```python
from build123d import *
from build123d.topology import SkipClean

# Parameters (mm, degrees)
SKETCH1_R           = 15.5
SKETCH1_R_2         = 12
BOSS_EXTRUDE1_DEPTH = 4
BOSS_EXTRUDE2_START = 13
SKETCH2_R           = 14
SKETCH2_R_2         = 12
BOSS_EXTRUDE2_DEPTH = 13
BOSS_EXTRUDE3_DEPTH = 0.5
CIRPATTERN1_COUNT   = 4
BOSS_EXTRUDE4_START = -4
SKETCH4_R           = 1.5
BOSS_EXTRUDE4_DEPTH = 4
CIRPATTERN2_COUNT   = 4
SKETCH5_R           = 12
BOSS_EXTRUDE5_DEPTH = 2


with BuildPart() as part:
    # Sketch1 → Boss-Extrude1 (new body)
    with BuildSketch(Plane(origin=(0, 0, 0), x_dir=(1, 0, 0), z_dir=(0, 1, 0))):
        with Locations(Location((0, 0, 0), (0, 0, 270))):
            Circle(SKETCH1_R)
        with Locations(Location((0, 0, 0), (0, 0, 270))):
            Circle(SKETCH1_R_2, mode=Mode.SUBTRACT)
    extrude(amount=BOSS_EXTRUDE1_DEPTH)

    # Sketch2 → Boss-Extrude2 (add)
    with SkipClean():  # the faces are left unmerged after this step: merging them gives an invalid solid
        with BuildSketch(Plane.XZ.offset(BOSS_EXTRUDE2_START)):
            with Locations(Location((0, 0, 0), (0, 0, 90))):
                Circle(SKETCH2_R)
            with Locations(Location((0, 0, 0), (0, 0, 270))):
                Circle(SKETCH2_R_2, mode=Mode.SUBTRACT)
        extrude(amount=-BOSS_EXTRUDE2_DEPTH)

    # Sketch3 → Boss-Extrude3 (add, symmetric)
    with SkipClean():  # the faces are left unmerged after this step: merging them gives an invalid solid
        with BuildSketch(Plane(origin=(0, 0, 0), x_dir=(0, 0, -1), z_dir=(1, 0, 0))):
            Polygon((-12, 0), (-3.5, -11), (3.5, -11), (12, 0), (12, -13), (-12, -13), align=None)
        boss_extrude3 = extrude(amount=BOSS_EXTRUDE3_DEPTH, both=True)

    # CirPattern1: Boss-Extrude3 ×4 about axis
    with SkipClean():  # the faces are left unmerged after this step: merging them gives an invalid solid
        cirpattern1_axis = Axis((0, 0, 0), (0, 1, 0))
        for i in range(1, CIRPATTERN1_COUNT):
            add(boss_extrude3.rotate(cirpattern1_axis, i * 360 / CIRPATTERN1_COUNT))

    # Sketch4 → Boss-Extrude4 (add)
    with SkipClean():  # the faces are left unmerged after this step: merging them gives an invalid solid
        with BuildSketch(Plane(origin=(0, 4, 0), x_dir=(1, 0, 0), z_dir=(0, 1, 0)).offset(BOSS_EXTRUDE4_START)):
            with BuildLine():
                Line((-2.785012774, 19.115214709), (-4.5, 14.832396974))
                ThreePointArc((-4.5, 14.832396974), (0, 15.5), (4.5, 14.832396974))
                Line((4.5, 14.832396974), (2.785012774, 19.115214709))
                ThreePointArc((2.785012774, 19.115214709), (0, 21), (-2.785012774, 19.115214709))
            make_face()
            with Locations(Location((0, 18, 0), (0, 0, 270))):
                Circle(SKETCH4_R, mode=Mode.SUBTRACT)
        boss_extrude4 = extrude(amount=BOSS_EXTRUDE4_DEPTH)

    # CirPattern2: Boss-Extrude4 ×4 about axis
    with SkipClean():  # the faces are left unmerged after this step: merging them gives an invalid solid
        cirpattern2_axis = Axis((0, 0, 0), (0, 1, 0))
        for i in range(1, CIRPATTERN2_COUNT):
            add(boss_extrude4.rotate(cirpattern2_axis, i * 360 / CIRPATTERN2_COUNT))

    # Sketch5 → Boss-Extrude5 (add)
    with SkipClean():  # the faces are left unmerged after this step: merging them gives an invalid solid
        with BuildSketch(Plane.XZ.offset(13)):
            with Locations(Location((0, 0, 0), (0, 0, 267.611984537))):
                Circle(SKETCH5_R)
        extrude(amount=-BOSS_EXTRUDE5_DEPTH)


solid = part.part
```
CAD build for the part. Positions are in the model's coordinates, mm. A direction names the side the tool comes from. Round coordinates to 2 decimals unless told otherwise and drop trailing zeros. Order: outer loops, then holes, each group sorted by start corner. A loop starts at its lowest first (then second) coordinate and runs counter-clockwise, first axis right, second up.
Q1. Slice it at B-B (z = 18.5). Write the cut outline in (x, y), and give its area (3 significant figures).
Q2. Slice it at A-A (y = 1.25). Write the cut outline in (x, z), and give its area (3 significant figures).
Q3. Drop flat-ended pins along their axis: pin 1 (2.5 mm diameter, centred on y = -3, z = -8, fed in from -X); pin 2 (7 mm diameter, centred on y = -6.5, z = 8.5, fed in from -X); pin 3 (2 mm diameter, centred on y = 1.5, z = -2, fed in from +X). Give the stop position or say it passes through.
Q4. Which spindle directions (+Z, -Z, +X, -X, +Y, -Y) get a long thin tool onto all of the face, cutting with end or side? Do faces 1 (the flat face through (17, 1.97, -3.63)), 2 (the flat face through (0.01, -5.58, -7.69)). Say none if no direction does.
Q5. Two-plate mould, pull along X, no slides. Class faces 3 (the cylindrical face through (-21, 2, 0)), 4 (the cylindrical face through (-0.07, 1.97, 19.5)), 5 (the flat face through (3.63, 1.97, 17)), 6 (the flat face through (0.01, -5.42, 7.81)): pulls with the +X half, pulls with the -X half, needs draft (parallel to the pull), parting line crosses it, or undercut.
Q6. Slice it at C-C (x = 18). Write the cut outline in (y, z).
Q7. Slice it at D-D (y = -4). Write the cut outline in (x, z).
Q8. Wall check: L1, parallel to Z at x = -3, y = -6.5; L2, parallel to Z at x = -8, y = -7; L3, parallel to Z at x = 18, y = 2.65. Give the ranges that are in metal, low to high.
Results below:
1. outline: (-3.03, 0) - (-1.41, 0) - (-1.41, 4) - (-3.03, 4) - close; (1.41, 0) - (3.03, 0) - (3.03, 4) - (1.41, 4) - close
1. area: 12.9 mm2
2. outline: (-19.12, -2.79) - (-14.83, -4.5) arc R15.5 ccw to (-4.5, -14.83) - (-2.79, -19.12) arc R3 ccw to (2.79, -19.12) - (4.5, -14.83) arc R15.5 ccw to (14.83, -4.5) - (19.12, -2.79) arc R3 ccw to (19.12, 2.79) - (14.83, 4.5) arc R15.5 ccw to (4.5, 14.83) - (2.79, 19.12) arc R3 ccw to (-2.79, 19.12) - (-4.5, 14.83) arc R15.5 ccw to (-14.83, 4.5) - (-19.12, 2.79) arc R3 ccw to start; hole circle Ø3 at (-18, 0); hole circle Ø24 at (0, 0); hole circle Ø3 at (0, -18); hole circle Ø3 at (0, 18); hole circle Ø3 at (18, 0)
2. area: 413 mm2
3. pin 1: stops at x = -12.27
3. pin 2: stops at x = -13.08
3. pin 3: stops at x = 20.83
4. face 1: -Z, +X, +Y, -Y
4. face 2: +Y
5. face 3: pulls with the -X half
5. face 4: undercut
5. face 5: pulls with the +X half
5. face 6: undercut
6. outline: (0, -3.23) - (4, -3.23) - (4, -1.5) - (0, -1.5) - close; (0, 1.5) - (4, 1.5) - (4, 3.23) - (0, 3.23) - close
7. outline: circle Ø28 at (0, 0); hole (-11.99, -0.5) arc R12 ccw to (-0.5, -11.99) - (-0.5, -8.91) - (0.5, -8.91) - (0.5, -11.99) arc R12 ccw to (11.99, -0.5) - (8.91, -0.5) - (8.91, 0.5) - (11.99, 0.5) arc R12 ccw to (0.5, 11.99) - (0.5, 8.91) - (-0.5, 8.91) - (-0.5, 11.99) arc R12 ccw to (-11.99, 0.5) - (-8.91, 0.5) - (-8.91, -0.5) - close
8. L1: z = -13.67 to -11.62, 11.62 to 13.67
8. L2: z = -11.49 to -8.94, -0.5 to 0.5, 8.94 to 11.49
8. L3: z = -3.23 to -1.5, 1.5 to 3.23
